from build123d import *

# Parameters (mm, degrees)
SKETCH1_R           = 1.5875
BOSS_EXTRUDE1_DEPTH = 6.35
BOSS_EXTRUDE2_START = 6.35
SKETCH1_4_R         = 1.5875
BOSS_EXTRUDE2_DEPTH = 3.302
SKETCH2_R           = 4.699
BOSS_EXTRUDE3_DEPTH = 3.175
CUT_EXTRUDE1_DEPTH  = 20.32
FILLET1_R           = 3.175


with BuildPart() as part:
    # Sketch1 → Boss-Extrude1 (new body)
    # profile 1 of 3: a face of its own
    with BuildSketch(Plane(origin=(0, 0, 0), x_dir=(1, 0, 0), z_dir=(0, 1, 0))):
        with BuildLine():
            Line((-12.7, -6.35), (12.7, -6.35))
            ThreePointArc((12.7, -6.35), (19.05, 0), (12.7, 6.35))
            Line((12.7, 6.35), (-12.7, 6.35))
            ThreePointArc((-12.7, 6.35), (-19.05, 0), (-12.7, -6.35))
        make_face()
        with Locations((-12.7, 0)):
            Circle(SKETCH1_R, mode=Mode.SUBTRACT)
        with Locations((12.7, 0)):
            Circle(SKETCH1_R, mode=Mode.SUBTRACT)
    # profile 2 of 3: a face of its own
    with BuildSketch(Plane(origin=(0, 0, 0), x_dir=(1, 0, 0), z_dir=(0, 1, 0))):
        with Locations((-12.7, 0)):
            Circle(SKETCH1_R)
    # profile 3 of 3: a face of its own
    with BuildSketch(Plane(origin=(0, 0, 0), x_dir=(1, 0, 0), z_dir=(0, 1, 0))):
        with Locations((12.7, 0)):
            Circle(SKETCH1_R)
    extrude(amount=BOSS_EXTRUDE1_DEPTH)

    # Sketch1<4> → Boss-Extrude2 (add)
    with BuildSketch(Plane(origin=(0, 0, 0), x_dir=(1, 0, 0), z_dir=(0, 1, 0)).offset(BOSS_EXTRUDE2_START)):
        with Locations(Location((-12.7, 0, 0), (0, 0, 90))):
            Circle(SKETCH1_4_R)
        with Locations(Location((12.7, 0, 0), (0, 0, 90))):
            Circle(SKETCH1_4_R)
    extrude(amount=BOSS_EXTRUDE2_DEPTH)

    # Sketch2 → Boss-Extrude3 (add)
    with BuildSketch(Plane(origin=(0, 9.652, 0), x_dir=(1, 0, 0), z_dir=(0, 1, 0))):
        with Locations(Location((-12.7, 0, 0), (0, 0, 270))):
            Circle(SKETCH2_R)
        with Locations(Location((12.7, 0, 0), (0, 0, 270))):
            Circle(SKETCH2_R)
    extrude(amount=BOSS_EXTRUDE3_DEPTH)

    # Sketch3 → Cut-Extrude1 (cut, symmetric)
    with BuildSketch(Plane(origin=(0, 0, 0), x_dir=(0, 0, -1), z_dir=(1, 0, 0))):
        with BuildLine():
            Line((6.35, 0), (6.35, 5.55625))
            ThreePointArc((6.35, 5.55625), (6.288919267, 5.120130209), (6.110377358, 4.717570755))
            ThreePointArc((6.110377358, 4.717570755), (5.697499195, 3.786652016), (5.55625, 2.778125))
            ThreePointArc((5.55625, 2.778125), (5.697499195, 1.769597984), (6.110377358, 0.838679245))
            ThreePointArc((6.110377358, 0.838679245), (6.288919267, 0.436119791), (6.35, 0))
        make_face()
        with BuildLine():
            ThreePointArc((-6.110377358, 4.717570755), (-6.288919267, 5.120130209), (-6.35, 5.55625))
            Line((-6.35, 5.55625), (-6.35, 0))
            ThreePointArc((-6.35, 0), (-6.288919267, 0.436119791), (-6.110377358, 0.838679245))
            ThreePointArc((-6.110377358, 0.838679245), (-5.697499195, 1.769597984), (-5.55625, 2.778125))
            ThreePointArc((-5.55625, 2.778125), (-5.697499195, 3.786652016), (-6.110377358, 4.717570755))
        make_face()
    extrude(amount=CUT_EXTRUDE1_DEPTH, both=True, mode=Mode.SUBTRACT)

    # Fillet1
    fillet1_edges = [part.edges().sort_by_distance(p)[0] for p in [
        (-12.7, 12.827, -4.699),
        (12.7, 12.827, -4.699),
    ]]
    fillet(fillet1_edges, radius=FILLET1_R - 0.0001)  # a hair under: the kernel refuses the full size


solid = part.part
Could you check a few things on this model? Use its own coordinates, in mm. A direction names the side the tool comes from. Give positions to 0.01 mm unless a question says otherwise; leave off trailing zeros. Order: outer loops, then holes, each group sorted by start corner. A loop starts at its lowest first (then second) coordinate and runs counter-clockwise, first axis right, second up. Notation, with made-up numbers: (-25, 60.25) - (19, 60.25) arc R28 cw to (19, 79.25) - close; hole circle Ø9 at (26.25, -23). An arc over 180 degrees is marked (long way). One line per item, written item: value. Start each with the question number.
1. Thinking about a two-plate mould opening in Y: for faces 1 (the face through (-13, 12.827, 0)), 2 (the face through (0.2, 0.4, 6.3)), 3 (the face through (0, 0, 0)), which applies, +Y half, -Y half, draft (parallel to the pull), parting line (faces both ways), or undercut?
2. If I drill on probe 1 along Y at (x, z) = (0.5, -4.25); probe 2 along Y at (x, z) = (9.5, -2.75); probe 3 along Y at (x, z) = (11, 2.5), over which ranges is the centre line in solid material (lowest first)?
3. Imagine slicing it at B-B on z = 2.75. Give the number of separate pieces and of enclosed holes in the cut face, plus the area to 3 significant figures.
4. Imagine slicing it at C-C on y = 4. List the corners of the cut face in (x, z) for me, plus the area to 3 significant figures.
5. For faces 4 (the face through (0.202, 5.114, 6.287)), 5 (the face through (-0.2, 5.13, -6.29)), 6 (the face through (-14.274, 7.978, 0.207)), which set-ups out of +Z, -Z, +X, -X, +Y, -Y let a thin tool reach every point of the face, with its end or its side?
6. For P1, Ø2, axis at x = 10, y = 1.5, coming from the +Z side; P2, Ø2, axis at y = 2.5, z = -4, coming from the -X side, each with a flat end and sliding along its axis, tell me the tip position at first contact or that it passes through.
Values:
1. face 1: +Y half
1. face 2: undercut
1. face 3: -Y half
2. probe 1: 0 to 6.35
2. probe 2: 0 to 6.35, 9.65 to 11.33
2. probe 3: 0 to 6.35, 9.65 to 12.45
3. separate pieces: 3
3. enclosed holes: 0
3. area: 270 mm²
4. outline: (-15.36, -5.77) - (15.36, -5.77) arc R6.35 ccw to (15.36, 5.77) - (-15.36, 5.77) arc R6.35 ccw to start
4. area: 415 mm²
5. face 4: +Z, +X, -X
5. face 5: -Z, +X, -X
5. face 6: none
6. P1: z = 6.27
6. P2: x = -18.3
